```python
from build123d import *

# Parameters (mm, degrees)
SKETCH2_R           = 2.159
SKETCH2_R_2         = 2.54
SKETCH2_R_3         = 1.25
BOSS_EXTRUDE1_DEPTH = 3.175


with BuildPart() as part:
    # Sketch2 → Boss-Extrude1 (new body)
    with BuildSketch(Plane(origin=(0, 0, 0), x_dir=(1, 0, 0), z_dir=(0, 1, 0))):
        Polygon((0, 10), (0, 244), (10, 254), (117, 254), (127, 244), (127, 10), (117, 0), (10, 0), align=None)
        with Locations(Location((6.35, 88.9, 0), (0, 0, 270))):
            Circle(SKETCH2_R, mode=Mode.SUBTRACT)
        with Locations(Location((6.35, 165.1, 0), (0, 0, 270))):
            Circle(SKETCH2_R, mode=Mode.SUBTRACT)
        with Locations(Location((120.65, 165.1, 0), (0, 0, 270))):
            Circle(SKETCH2_R, mode=Mode.SUBTRACT)
        with Locations(Location((120.81, 50.8, 0), (0, 0, 270))):
            Circle(SKETCH2_R, mode=Mode.SUBTRACT)
        with Locations(Location((6.35, 50.8, 0), (0, 0, 270))):
            Circle(SKETCH2_R, mode=Mode.SUBTRACT)
        with Locations(Location((25.4, 247.65, 0), (0, 0, 270))):
            Circle(SKETCH2_R, mode=Mode.SUBTRACT)
        with Locations(Location((101.6, 247.65, 0), (0, 0, 270))):
            Circle(SKETCH2_R, mode=Mode.SUBTRACT)
        with Locations(Location((101.6, 6.35, 0), (0, 0, 270))):
            Circle(SKETCH2_R, mode=Mode.SUBTRACT)
        with Locations(Location((25.4, 6.35, 0), (0, 0, 270))):
            Circle(SKETCH2_R, mode=Mode.SUBTRACT)
        with Locations(Location((15.621, 241.3, 0), (0, 0, 270))):
            Circle(SKETCH2_R, mode=Mode.SUBTRACT)
        with Locations(Location((15.621, 199.39, 0), (0, 0, 270))):
            Circle(SKETCH2_R, mode=Mode.SUBTRACT)
        with Locations(Location((111.379, 199.39, 0), (0, 0, 270))):
            Circle(SKETCH2_R, mode=Mode.SUBTRACT)
        with Locations(Location((111.379, 241.3, 0), (0, 0, 270))):
            Circle(SKETCH2_R, mode=Mode.SUBTRACT)
        with Locations(Location((46.355, 169.545, 0), (0, 0, 270))):
            Circle(SKETCH2_R, mode=Mode.SUBTRACT)
        with Locations(Location((46.355, 84.455, 0), (0, 0, 270))):
            Circle(SKETCH2_R, mode=Mode.SUBTRACT)
        with Locations(Location((80.645, 84.455, 0), (0, 0, 270))):
            Circle(SKETCH2_R, mode=Mode.SUBTRACT)
        with Locations(Location((80.645, 169.545, 0), (0, 0, 270))):
            Circle(SKETCH2_R, mode=Mode.SUBTRACT)
        with Locations(Location((120.65, 88.9, 0), (0, 0, 270))):
            Circle(SKETCH2_R, mode=Mode.SUBTRACT)
        with Locations(Location((48.50003, 234.95, 0), (0, 0, 270))):
            Circle(SKETCH2_R_2, mode=Mode.SUBTRACT)
        with Locations(Location((78.49997, 234.95, 0), (0, 0, 270))):
            Circle(SKETCH2_R_2, mode=Mode.SUBTRACT)
        with Locations(Location((78.49997, 204.95006, 0), (0, 0, 270))):
            Circle(SKETCH2_R_2, mode=Mode.SUBTRACT)
        with Locations(Location((48.50003, 204.95006, 0), (0, 0, 270))):
            Circle(SKETCH2_R_2, mode=Mode.SUBTRACT)
        with Locations(Location((120.65, 203.2, 0), (0, 0, 270))):
            Circle(SKETCH2_R, mode=Mode.SUBTRACT)
        with Locations(Location((6.35, 203.2, 0), (0, 0, 270))):
            Circle(SKETCH2_R, mode=Mode.SUBTRACT)
        with Locations(Location((63.5, 247.65, 0), (0, 0, 270))):
            Circle(SKETCH2_R, mode=Mode.SUBTRACT)
        with Locations(Location((63.5, 6.35, 0), (0, 0, 270))):
            Circle(SKETCH2_R, mode=Mode.SUBTRACT)
        with Locations(Location((120.65, 127, 0), (0, 0, 270))):
            Circle(SKETCH2_R, mode=Mode.SUBTRACT)
        with Locations(Location((6.35, 127, 0), (0, 0, 270))):
            Circle(SKETCH2_R, mode=Mode.SUBTRACT)
        with Locations(Location((25.4, 45.4, 0), (0, 0, 270))):
            Circle(SKETCH2_R_3, mode=Mode.SUBTRACT)
        with Locations(Location((45.4, 65.4, 0), (0, 0, 270))):
            Circle(SKETCH2_R_3, mode=Mode.SUBTRACT)
        with Locations(Location((45.4, 25.4, 0), (0, 0, 270))):
            Circle(SKETCH2_R_3, mode=Mode.SUBTRACT)
        with BuildLine():
            Line((34.808835003, 152.4), (34.808835003, 101.6))
            ThreePointArc((34.808835003, 101.6), (31.633835003, 98.425), (28.458835003, 101.6))
            Line((28.458835003, 101.6), (28.458835003, 152.4))
            ThreePointArc((28.458835003, 152.4), (31.633835003, 155.575), (34.808835003, 152.4))
        make_face(mode=Mode.SUBTRACT)
        with BuildLine():
            Line((92.191164997, 152.4), (92.191164997, 101.6))
            ThreePointArc((92.191164997, 101.6), (95.366164997, 98.425), (98.541164997, 101.6))
            Line((98.541164997, 101.6), (98.541164997, 152.4))
            ThreePointArc((98.541164997, 152.4), (95.366164997, 155.575), (92.191164997, 152.4))
        make_face(mode=Mode.SUBTRACT)
    extrude(amount=BOSS_EXTRUDE1_DEPTH)


solid = part.part
```
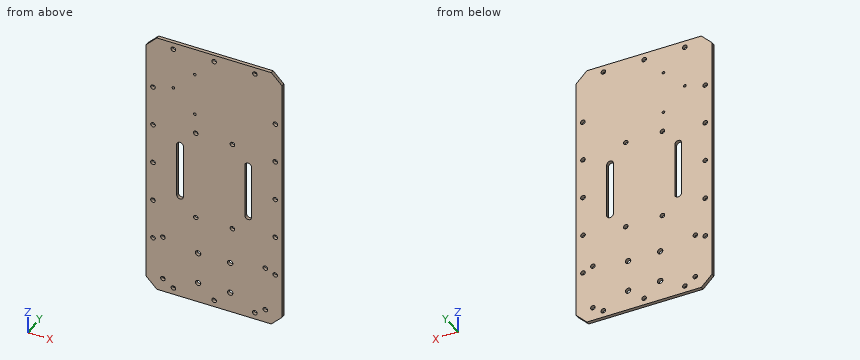
Source: CAD feature listing. Evaluate the final solid. Frame: model axes, mm. Give positions to 0.01 mm unless a question says otherwise; leave off trailing zeros. Loops run counter-clockwise (first coordinate to the right, second up) from the corner with the lowest first, then second, coordinate; pieces in that order, holes last. Notation, with made-up numbers: (33, 33) -> (62, 33) arc R28 ccw to (62, 52) -> close; hole circle Ø5 at (23.25, 24). An arc over 180 degrees is marked (long way). Put each result on its own line as item: value. Start each with the question number.
1) Material intervals for probe 1 along X at (y, z) = (1.85, -241.3); probe 2 along X at (y, z) = (2.3, -150.5); probe 3 along Z at (x, y) = (49, 2.85), sorted ascending.
2) Cut plane B-B (y = 1.25). State how many separate pieces and enclosed holes the cut face has, then the cut area to 3 significant figures.
3) Cut plane A-A (z = -147). Return loops of the section in (x, y) (3 decimals), then the cut area to 3 significant figures.
4) Contact query for a flat-ended pin moving along its axis: P1, Ø3, axis at x = 48.5, z = -204.95, coming from the -Y side. Output: stop coordinate, or through.
Results are:
1. probe 1: x = 0 to 13.46, 17.78 to 109.22, 113.54 to 127
1. probe 2: x = 0 to 28.46, 34.81 to 92.19, 98.54 to 127
1. probe 3: z = -254 to -237.44, -232.46 to -207.44, -202.46 to 0
2. separate pieces: 1
2. enclosed holes: 33
2. area: 30,900 mm2
3. outline: (0, 0) -> (28.459, 0) -> (28.459, 3.175) -> (0, 3.175) -> close; (34.809, 0) -> (92.191, 0) -> (92.191, 3.175) -> (34.809, 3.175) -> close; (98.541, 0) -> (127, 0) -> (127, 3.175) -> (98.541, 3.175) -> close
3. area: 363 mm2
4. P1: passes through
